from build123d import *

# Parameters (mm, degrees)
SKETCH_1_W          = 40
SKETCH_1_H          = 3
EXTRUDE_1_DEPTH     = 20
SKETCH_2_R          = 2.25
CUT_EXTRUDE_1_DEPTH = 2
SKETCH_3_R          = 3.75
CUT_EXTRUDE_2_DEPTH = 3
CUT_EXTRUDE_3_DEPTH = 3
SKETCH_5_W          = 10
SKETCH_5_H          = 12
CUT_EXTRUDE_4_DEPTH = 12
CUT_EXTRUDE_5_DEPTH = 30


with BuildPart() as part:
    # 草图1 → 凸台-拉伸1 (new body)
    with BuildSketch(Plane.XY):
        with BuildLine():
            ThreePointArc((0, -1.65), (-1.166726189, 1.166726189), (1.65, 0))
            Line((1.65, 0), (6, 0))
            ThreePointArc((6, 0), (-4.242640687, 4.242640687), (0, -6))
            Line((0, -6), (0, -1.65))
        make_face()
        with BuildLine():
            Line((6, 0), (1.65, 0))
            ThreePointArc((1.65, 0), (1.166726189, -1.166726189), (0, -1.65))
            Line((0, -1.65), (0, -6))
            ThreePointArc((0, -6), (4.242640687, -4.242640687), (6, 0))
        make_face()
        with BuildLine():
            Line((6, -15), (6, 0))
            ThreePointArc((6, 0), (4.242640687, -4.242640687), (0, -6))
            Line((0, -6), (0, -48))
            Line((0, -48), (6, -48))
            Line((6, -48), (6, -18))
            Line((6, -18), (6, -15))
        make_face()
        with Locations((26, -16.5)):
            Rectangle(SKETCH_1_W, SKETCH_1_H)
    extrude(amount=EXTRUDE_1_DEPTH)

    # 草图2 → 切除-拉伸1 (cut)
    with BuildSketch(Plane(origin=(0, -15, 0), x_dir=(1, 0, 0), z_dir=(0, 1, 0))):
        with BuildLine():
            ThreePointArc((37.2109375, -12.436802432), (34.75, -10.196711949), (37.2109375, -7.956621466))
            Line((37.2109375, -7.956621466), (21.3515625, -6.463227811))
            ThreePointArc((21.3515625, -6.463227811), (23.773162398, -7.672415946), (24.75, -10.196711949))
            ThreePointArc((24.75, -10.196711949), (23.773162398, -12.721007952), (21.3515625, -13.930196087))
            Line((21.3515625, -13.930196087), (37.2109375, -12.436802432))
        make_face()
        with Locations((37, -10.196711949)):
            Circle(SKETCH_2_R)
    extrude(amount=-CUT_EXTRUDE_1_DEPTH, mode=Mode.SUBTRACT)

    # 草图3 → 切除-拉伸2 (cut)
    with BuildSketch(Plane(origin=(0, -15, 0), x_dir=(1, 0, 0), z_dir=(0, 1, 0))):
        with Locations(Location((21, -10.196711949, 0), (0, 0, 180))):
            Circle(SKETCH_3_R)
    extrude(amount=-CUT_EXTRUDE_2_DEPTH, mode=Mode.SUBTRACT)

    # 草图4 → 切除-拉伸3 (cut)
    with BuildSketch(Plane(origin=(0, -17, 0), x_dir=(1, 0, 0), z_dir=(0, 1, 0))):
        with BuildLine():
            Line((28, -9.196711949), (37, -9.196711949))
            ThreePointArc((37, -9.196711949), (38, -10.196711949), (37, -11.196711949))
            Line((37, -11.196711949), (28, -11.196711949))
            ThreePointArc((28, -11.196711949), (27, -10.196711949), (28, -9.196711949))
        make_face()
    extrude(amount=-CUT_EXTRUDE_3_DEPTH, mode=Mode.SUBTRACT)

    # 草图5 → 切除-拉伸4 (cut)
    with BuildSketch(Plane(origin=(6, 0, 0), x_dir=(0, 0, -1), z_dir=(1, 0, 0))):
        with Locations((-10, 0)):
            Rectangle(SKETCH_5_W, SKETCH_5_H)
    extrude(amount=-CUT_EXTRUDE_4_DEPTH, mode=Mode.SUBTRACT)

    # 草图6 → 切除-拉伸5 (cut)
    with BuildSketch(Plane.XZ.offset(48)):
        with BuildLine():
            Line((6, 20), (6, 0))
            ThreePointArc((6, 0), (2.981888497, 10), (6, 20))
        make_face()
    extrude(amount=-CUT_EXTRUDE_5_DEPTH, mode=Mode.SUBTRACT)


solid = part.part
CAD build for the part. Positions are in the model's coordinates, mm. A direction names the side the tool comes from. Give positions to 0.01 mm unless a question says otherwise; leave off trailing zeros. Write each loop counter-clockwise with the first axis right and the second up, starting at its lowest first coordinate (ties: lowest second). Pieces come first, ordered by that corner, then holes. Notation, with made-up numbers: (-15, 13.25) - (40, 13.25) arc R13 ccw to (40, 24.25) - close; hole circle Ø1 at (-38.5, 66). An arc over 180 degrees is marked (long way). Put each result on its own line as item: value.
(1) Saw through at C-C (x = 4). List the corners of the cut face in (y, z).
Working result:
outline: (-48, 0) - (4.47, 0) - (4.47, 5) - (-6, 5) - (-6, 15) - (4.47, 15) - (4.47, 20) - (-48, 20) - (-48, 15.98) - (-18, 15.98) - (-18, 4.02) - (-48, 4.02) - close
(2) Wall check: L1, parallel to Z at x = 21, y = -15.55; L2, parallel to X at y = -7, z = 5.25; L3, parallel to Y at x = 32, z = 15.5. Give the ranges that are in metal, low to high.
Working result:
L1: 0 to 6.45, 13.95 to 20
L2: 0 to 6
L3: -18 to -15
(3) Drop flat-ended pins along their axis: pin 1 Ø1 at (x, z) = (11, 15.5) entering from -Y; pin 2 Ø1 at (x, z) = (29, 18) entering from +Y; pin 3 Ø3 at (x, z) = (3.5, 8.5) entering from +Y. Give the stop position or say it passes through.
Working result:
pin 1: y = -18
pin 2: y = -15
pin 3: y = -6
(4) Saw through at D-D (y = -11.5). List the corners of the cut face in (x, z).
Working result:
outline: (0, 0) - (6, 0) - (6, 20) - (0, 20) - close
(5) Tool access for faces 1 (the flat face through (0, -27, 10)), 2 (the flat face through (6, -9, 10)), 3 (the cylindrical face through (2.982, -33.21, 9.852)): list every direction of +Z, -Z, +X, -X, +Y, -Y with a clear straight run to the whole face (end or side of a thin tool).
Working result:
face 1: +Z, -Z, -X, -Y
face 2: +Z, -Z, +X, +Y
face 3: +X, -Y
(6) Saw through at B-B (y = 2.5). List the corners of the cut face in (x, z).
Working result:
outline: (-5.45, 0) - (5.45, 0) - (5.45, 5) - (-5.45, 5) - close; (-5.45, 15) - (5.45, 15) - (5.45, 20) - (-5.45, 20) - close
(7) Pull direction Z, two halves, no side cores. Call faces 4 (the cylindrical face through (-4.1, 4.38, 17.46)), 5 (the flat face through (1.4, -1.4, 5)), 6 (the flat face through (1.4, -1.4, 15)), 7 (the flat face through (6, -17, 20)): released by +Z, released by -Z, zero draft, split by the parting line, or undercut.
Working result:
face 4: zero draft
face 5: undercut
face 6: undercut
face 7: released by +Z
(8) Saw through at A-A (z = 3.5). List the corners of the cut face in (x, y), then the cut area to 3 significant figures.
Working result:
outline: (0, -48) - (4.19, -48) - (4.19, -18) - (46, -18) - (46, -15) - (6, -15) - (6, 0) arc R6 ccw (long way) to (0, -6) - close; hole circle Ø3.3 at (0, 0)
area: 430 mm^2
